Design review of the part shown in the three views and the two pictorial views. Dimensions are in mm from the part's minimum x, y and z. Coordinates: 2 decimals unless noted, no trailing zeros. Loops run counter-clockwise (first coordinate to the right, second up) from the corner with the lowest first, then second, coordinate; pieces in that order, holes last. Notation, with made-up numbers: (-24, 28) - (34, 28) arc R27 cw to (34, 51) - close; hole circle Ø11 at (81, 29). An arc over 180 degrees is marked (long way). One line per item, written item: value. Start each with the question number.
1. To check wall thickness, follow line 1 (X direction, y = 17.5, z = 3.45); line 2 (Y direction, x = 39.5, z = 0.4); line 3 (X direction, y = 16.5, z = 3.3). State the ranges of each line that lie inside material, in increasing order. Write a range as from..to.
2. Take a section at C-C, the plane z = 3.35. State the section outline as (x, y) points.
3. Insertion check: pin 1 (6 mm diameter, centred on x = 39, y = 17.5, fed in from +Z); pin 2 (3.5 mm diameter, centred on x = 9.5, y = 17.5, fed in from +Z); pin 3 (1.8 mm diameter, centred on x = 9.5, y = 17.5, fed in from +Z). Each pin has a flat end and moves straight along its axis. Give the tip position at first contact, or say it passes through.
4. Take a section at B-B, the plane x = 9.5. State the section outline as (y, z) points.
5. Take a section at A-A, the plane y = 17.5. State the section outline as (x, z) points.
6. Take a section at D-D, the plane x = 40.5. State the section outline as (y, z) points.
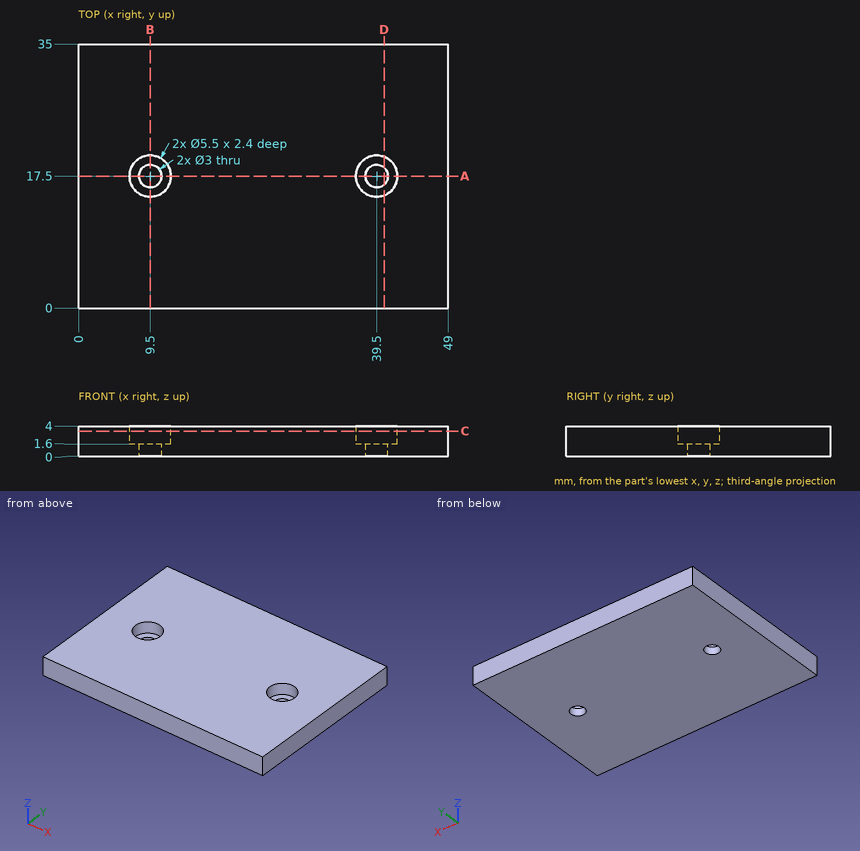
Solutions:
1. line 1: 0..6.75, 12.25..36.75, 42.25..49
1. line 2: 0..16, 19..35
1. line 3: 0..6.94, 12.06..36.94, 42.06..49
2. outline: (0, 0) - (49, 0) - (49, 35) - (0, 35) - close; hole circle Ø5.5 at (9.5, 17.5); hole circle Ø5.5 at (39.5, 17.5)
3. pin 1: z = 4
3. pin 2: z = 1.6
3. pin 3: through
4. outline: (0, 0) - (16, 0) - (16, 1.6) - (14.75, 1.6) - (14.75, 4) - (0, 4) - close; (19, 0) - (35, 0) - (35, 4) - (20.25, 4) - (20.25, 1.6) - (19, 1.6) - close
5. outline: (0, 0) - (8, 0) - (8, 1.6) - (6.75, 1.6) - (6.75, 4) - (0, 4) - close; (11, 0) - (38, 0) - (38, 1.6) - (36.75, 1.6) - (36.75, 4) - (12.25, 4) - (12.25, 1.6) - (11, 1.6) - close; (41, 0) - (49, 0) - (49, 4) - (42.25, 4) - (42.25, 1.6) - (41, 1.6) - close
6. outline: (0, 0) - (16.38, 0) - (16.38, 1.6) - (14.94, 1.6) - (14.94, 4) - (0, 4) - close; (18.62, 0) - (35, 0) - (35, 4) - (20.06, 4) - (20.06, 1.6) - (18.62, 1.6) - close
